For this review, take the finished solid that the model builds, in its own axes (mm). Face numbers are marked on the shaded views. A direction names the side the tool comes from. Round coordinates to 2 decimals unless told otherwise and drop trailing zeros. Order: outer loops, then holes, each group sorted by start corner. A loop starts at its lowest first (then second) coordinate and runs counter-clockwise, first axis right, second up. Notation, with made-up numbers: M -19.5,33 L -12.5,33 A22 ccw -12.5,66 Z; hole C 34.5,2 d1. An arc over 180 degrees is marked long. Put each result on its own line as item: value.
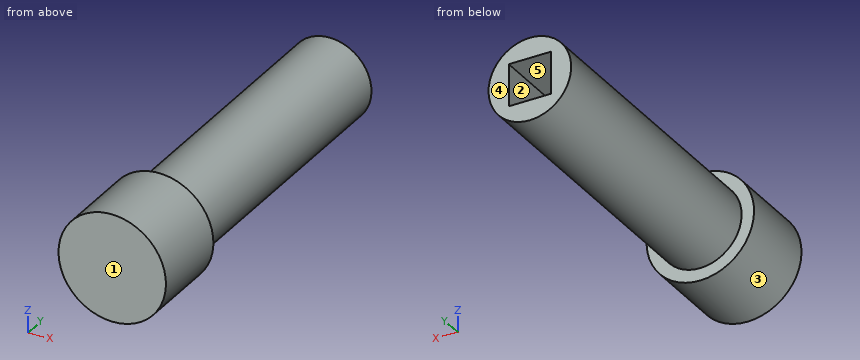
from build123d import *

# Parameters (mm, degrees)
SKETCH1_R           = 5
BOSS_EXTRUDE1_DEPTH = 45
SKETCH2_W           = 5.1
SKETCH2_H           = 5.1
CUT_EXTRUDE1_DEPTH  = 22
SKETCH3_R           = 6.5
BOSS_EXTRUDE2_DEPTH = 9.8


with BuildPart() as part:
    # Sketch1 → Boss-Extrude1 (new body)
    with BuildSketch(Plane(origin=(0, 0, 0), x_dir=(1, 0, 0), z_dir=(0, 1, 0))):
        with Locations(Location((0, 0, 0), (0, 0, 90))):
            Circle(SKETCH1_R)
    extrude(amount=BOSS_EXTRUDE1_DEPTH)

    # Sketch2 → Cut-Extrude1 (cut)
    with BuildSketch(Plane(origin=(0, 45, 0), x_dir=(1, 0, 0), z_dir=(0, 1, 0))):
        Rectangle(SKETCH2_W, SKETCH2_H)
    extrude(amount=-CUT_EXTRUDE1_DEPTH, mode=Mode.SUBTRACT)

    # Sketch3 → Boss-Extrude2 (add)
    with BuildSketch(Plane.XZ):
        with Locations(Location((0, 0, 0), (0, 0, 270))):
            Circle(SKETCH3_R)
    extrude(amount=-BOSS_EXTRUDE2_DEPTH)


solid = part.part
(1) To check wall thickness, follow L1, parallel to Y at x = 2.25, z = 2.5; L2, parallel to Y at x = -5, z = 4; L3, parallel to X at y = 43.5, z = 1.75. State the ranges of each line that lie inside material, in increasing order.
A:
L1: y = 0 to 23
L2: y = 0 to 9.8
L3: x = -4.68 to -2.55, 2.55 to 4.68
(2) Add section D-D on z = 4.5. Give the boundary of the cut face in (x, y).
A:
outline: M -4.69,0 L 4.69,0 L 4.69,9.8 L 2.18,9.8 L 2.18,45 L -2.18,45 L -2.18,9.8 L -4.69,9.8 Z
(3) For the marked faces 1 and 2, list the 3-axis set-ups (+Z, -Z, +X, -X, +Y, -Y) from which the entire face can be reached by the end or side of a thin tool; tool diameter is ignored.
A:
face 1: +Z, -Z, +X, -X, -Y
face 2: +Y
(4) Add section C-C on y = 16. Give the boundary of the cut face in (x, z), then the cut area to 3 significant figures.
A:
outline: C 0,0 d10
area: 78.5 mm2
(5) Add section B-B on z = 0. Give the boundary of the cut face in (x, y), then the cut area to 3 significant figures.
A:
outline: M -6.5,0 L 6.5,0 L 6.5,9.8 L 5,9.8 L 5,45 L 2.55,45 L 2.55,23 L -2.55,23 L -2.55,45 L -5,45 L -5,9.8 L -6.5,9.8 Z
area: 367 mm2
(6) Add section A-A on x = 0. Give the boundary of the cut face in (y, z).
A:
outline: M 0,-6.5 L 9.8,-6.5 L 9.8,-5 L 45,-5 L 45,-2.55 L 23,-2.55 L 23,2.55 L 45,2.55 L 45,5 L 9.8,5 L 9.8,6.5 L 0,6.5 Z
(7) Insertion check: pin 1 Ø4 at (y, z) = (30.5, 0.5) entering from -X; pin 2 Ø2.5 at (x, y) = (-1, 32) entering from +Z; pin 3 Ø1.5 at (y, z) = (33.5, 1) entering from +X. Each pin has a flat end and moves straight along its axis. Give the tip position at first contact, or say it passes through.
A:
pin 1: stops at x = -5
pin 2: stops at z = 5
pin 3: stops at x = 4.99
(8) Draft analysis for pull direction X (two halves, no side actions). For the marked faces 3, 4 and 5, state which applies: released by +X, released by -X, zero draft, split by the parting line, or undercut.
A:
face 3: split by the parting line
face 4: zero draft
face 5: undercut
